Source: CAD feature listing. Evaluate the final solid. Frame: model axes, mm. Round coordinates to 2 decimals unless told otherwise and drop trailing zeros. Loops run counter-clockwise (first coordinate to the right, second up) from the corner with the lowest first, then second, coordinate; pieces in that order, holes last. Notation, with made-up numbers: (-36.5, -26) -> (-23.5, -26) arc R27 cw to (-23.5, 7) -> close; hole circle Ø4 at (-12, -23.75). An arc over 180 degrees is marked (long way). Return JSON: item names as keys, results as strings. Group by question number.
```python
from build123d import *

# Parameters (mm, degrees)
SKETCH_1_W          = 90
SKETCH_1_H          = 28
SKETCH_1_R          = 4.25
SKETCH_1_R_2        = 2
EXTRUDE_1_DEPTH     = 3
CUT_EXTRUDE_1_REACH = 49.223
SKETCH_3_R          = 2.25
FILLET_1_RADIUS     = 14
FILLET_1_LENGTH     = 3
FILLET_2_RADIUS     = 14
FILLET_2_LENGTH     = 3


with BuildPart() as part:
    # 草图1 → 凸台-拉伸1 (new body)
    with BuildSketch(Plane(origin=(0, 0, 0), x_dir=(1, 0, 0), z_dir=(0, 1, 0))):
        Rectangle(SKETCH_1_W, SKETCH_1_H)
        with Locations(Location((17.5, 0, 0), (0, 0, 270))):
            Circle(SKETCH_1_R, mode=Mode.SUBTRACT)
        with Locations(Location((-32.5, 0, 0), (0, 0, 270))):
            Circle(SKETCH_1_R_2, mode=Mode.SUBTRACT)
    extrude(amount=EXTRUDE_1_DEPTH)

    # 草图3 → 切除-拉伸1 (cut, up to next)
    with BuildSketch(Plane(origin=(0, 3, 0), x_dir=(1, 0, 0), z_dir=(0, 1, 0)), mode=Mode.PRIVATE) as cut_extrude_1_sk1:
        with Locations(Location((36, 0, 0), (0, 0, 270))):
            Circle(SKETCH_3_R)
    cut_extrude_1_tool1 = extrude(cut_extrude_1_sk1.sketch, amount=-CUT_EXTRUDE_1_REACH, mode=Mode.PRIVATE) & part.part
    # 草图3 → 切除-拉伸1 (cut, up to next)
    with BuildSketch(Plane(origin=(0, 3, 0), x_dir=(1, 0, 0), z_dir=(0, 1, 0)), mode=Mode.PRIVATE) as cut_extrude_1_sk2:
        with Locations(Location((-1, 0, 0), (0, 0, 270))):
            Circle(SKETCH_3_R)
    cut_extrude_1_tool2 = extrude(cut_extrude_1_sk2.sketch, amount=-CUT_EXTRUDE_1_REACH, mode=Mode.PRIVATE) & part.part
    add(cut_extrude_1_tool1.solids().sort_by_distance((36, 3, 0))[0], mode=Mode.SUBTRACT)
    add(cut_extrude_1_tool2.solids().sort_by_distance((-1, 3, 0))[0], mode=Mode.SUBTRACT)

    # 圆角1: full round fillet: the end face becomes a half cylinder, R = half its width
    fillet_1_face = Plane((-45, 1.5, 0), x_dir=(0, 1, 0), z_dir=(-1, 0, 0))  # on the end face: x along it, z out of the body
    fillet_1_slab = fillet_1_face.offset(-FILLET_1_RADIUS / 2) * Box(FILLET_1_LENGTH, 2 * FILLET_1_RADIUS, FILLET_1_RADIUS, mode=Mode.PRIVATE)  # the body's end, R deep
    fillet_1_round = Plane((-31, 1.5, 0), x_dir=(-1, 0, 0), z_dir=(0, 1, 0)) * Cylinder(FILLET_1_RADIUS, FILLET_1_LENGTH, mode=Mode.PRIVATE)  # its axis R under the face
    add(fillet_1_slab - fillet_1_round, mode=Mode.SUBTRACT)

    # 圆角2: full round fillet: the end face becomes a half cylinder, R = half its width
    fillet_2_face = Plane((45, 1.5, 0), x_dir=(0, -1, 0), z_dir=(1, 0, 0))  # on the end face: x along it, z out of the body
    fillet_2_slab = fillet_2_face.offset(-FILLET_2_RADIUS / 2) * Box(FILLET_2_LENGTH, 2 * FILLET_2_RADIUS, FILLET_2_RADIUS, mode=Mode.PRIVATE)  # the body's end, R deep
    fillet_2_round = Plane((31, 1.5, 0), x_dir=(1, 0, 0), z_dir=(0, -1, 0)) * Cylinder(FILLET_2_RADIUS, FILLET_2_LENGTH, mode=Mode.PRIVATE)  # its axis R under the face
    add(fillet_2_slab - fillet_2_round, mode=Mode.SUBTRACT)


solid = part.part
```
(1) Mould query, pull axis Z, two halves, no side actions, for faces 1 (the face through (0, 1, -14)), 2 (the face through (38.23, 1.52, -0.29)), 3 (the face through (-34.452, 1.479, -0.434)), 4 (the face through (-1, 3, -3)). Classes: released by +Z, released by -Z, zero draft, split by the parting line, or undercut.
(2) Pin query (flat end, axial travel): pin 1 (8 mm diameter, centred on x = -14.5, z = 4.5, fed in from -Y); pin 2 (1.5 mm diameter, centred on y = 2, z = 4.5, fed in from +X). Return the tip coordinate at first contact, or that it passes through.
(3) Cut plane B-B (z = 0). Return loops of the section in (x, y).
(4) Ray query, line 1 (X direction, y = 0.8, z = 0); line 2 (X direction, y = 1.05, z = 1.5); line 3 (X direction, y = 2.5, z = -3). Return the intervals inside material, ascending.
(5) Cut plane D-D (x = 17.5). Return loops of the section in (y, z), and give its area (3 significant figures).
(6) Cut plane A-A (x = -1). Return loops of the section in (y, z).
(7) Cut plane C-C (y = 1). Return loops of the section in (x, z).
Answers follow:
{
 "1": {"face 1": "released by -Z", "face 2": "undercut", "face 3": "undercut", "face 4": "zero draft"},
 "2": {"pin 1": "y = 0", "pin 2": "x = 44.49"},
 "3": {"outline": "(-45, 0) -> (-34.5, 0) -> (-34.5, 3) -> (-45, 3) -> close; (-30.5, 0) -> (-3.25, 0) -> (-3.25, 3) -> (-30.5, 3) -> close; (1.25, 0) -> (13.25, 0) -> (13.25, 3) -> (1.25, 3) -> close; (21.75, 0) -> (33.75, 0) -> (33.75, 3) -> (21.75, 3) -> close; (38.25, 0) -> (45, 0) -> (45, 3) -> (38.25, 3) -> close"},
 "4": {"line 1": "-45 to -34.5, -30.5 to -3.25, 1.25 to 13.25, 21.75 to 33.75, 38.25 to 45", "line 2": "-44.92 to -33.82, -31.18 to -2.68, 0.68 to 13.52, 21.48 to 34.32, 37.68 to 44.92", "line 3": "-44.67 to 14.49, 20.51 to 44.67"},
 "5": {"outline": "(0, -14) -> (3, -14) -> (3, -4.25) -> (0, -4.25) -> close; (0, 4.25) -> (3, 4.25) -> (3, 14) -> (0, 14) -> close", "area": "58.5 mm^2"},
 "6": {"outline": "(0, -14) -> (3, -14) -> (3, -2.25) -> (0, -2.25) -> close; (0, 2.25) -> (3, 2.25) -> (3, 14) -> (0, 14) -> close"},
 "7": {"outline": "(-31, -14) -> (31, -14) arc R14 ccw to (31, 14) -> (-31, 14) arc R14 ccw to start; hole circle Ø4 at (-32.5, 0); hole circle Ø4.5 at (-1, 0); hole circle Ø8.5 at (17.5, 0); hole circle Ø4.5 at (36, 0)"}
}
